Autodesk Inventor part; units mm, degrees
ref_plane "YZ Plane" through (0, 0, 0) normal (1, 0, 0) x (0, 1, 0)
ref_plane "XZ Plane" through (0, 0, 0) normal (0, 1, 0) x (-1, 0, 0)
ref_plane "XY Plane" through (0, 0, 0) normal (0, 0, 1) x (1, 0, 0)
sketch "Boceto1" plane through (0, 0, 0) normal (0, 1, 0) x (-1, 0, 0)
  line L0 (0, 0) -> (0, -2.6)
  line L1 (0, -2.6) -> (-2.7, -2.6)
  line L2 (-2.7, -2.6) -> (-2.7, -5.7)
  line L3 (-2.7, -5.7) -> (-12, -5.7)
  line L4 (-12, -5.7) -> (-12, -2.6)
  line L5 (-12, -2.6) -> (-14.7, -2.6)
  line L6 (-14.7, -2.6) -> (-14.7, 0)
  line L7 (-14.7, 0) -> (0, 0)
  line L8 (-12, -5.7) -> (-11.9, -5.7)
  line L9 (-11.9, -5.7) -> (-11.9, -2.6)
  line L10 (-11.9, -2.6) -> (-12, -2.6)
  line L11 (-12, -2.6) -> (-12, -5.7)
  line L12 (-2.7, -5.7) -> (-2.8, -5.7)
  line L13 (-2.8, -5.7) -> (-2.8, -2.6)
  line L14 (-2.8, -2.6) -> (-2.7, -2.6)
  line L15 (-2.7, -2.6) -> (-2.7, -5.7)
  line L16 (-2.7, -5.7) -> (4.75, -5.7)
  line L17 (-2.7, -5.7) -> (4.75, -5.7) construction
  line L18 (-12, -5.7) -> (-19.45, -5.7)
  line L19 (-12, -5.7) -> (-4.55, -5.7) construction
  line L20 (4.75, -5.7) -> (5.75, -5.7)
  line L21 (7.75, -7.7) -> (7.75, -8.7)
  line L22 (7.75, -8.7) -> (4.75, -8.7)
  line L23 (4.75, -8.7) -> (4.75, -5.7)
  line L24 (-19.45, -5.7) -> (-20.45, -5.7)
  line L25 (-22.45, -7.7) -> (-22.45, -8.7)
  line L26 (-22.45, -8.7) -> (-19.45, -8.7)
  line L27 (-19.45, -8.7) -> (-19.45, -5.7)
  line L28 (4.75, -8.7) -> (-19.45, -8.7)
  line L29 (4.75, -8.7) -> (7.75, -8.7)
  line L30 (7.75, -8.7) -> (7.75, -27.1)
  line L31 (7.75, -27.1) -> (4.75, -27.1)
  line L32 (4.75, -27.1) -> (4.75, -8.7)
  line L33 (-22.45, -8.7) -> (-19.45, -8.7)
  line L34 (-19.45, -8.7) -> (-19.45, -27.1)
  line L35 (-19.45, -27.1) -> (-22.45, -27.1)
  line L36 (-22.45, -27.1) -> (-22.45, -8.7)
  line L37 (7.75, -27.1) -> (-22.45, -27.1)
  line L38 (-22.45, -27.1) -> (-22.45, -28.1)
  line L39 (-20.45, -30.1) -> (5.75, -30.1)
  line L40 (7.75, -28.1) -> (7.75, -27.1)
  arc A0 (7.75, -7.7) -> (5.75, -5.7) centre (5.75, -7.7) ccw
  arc A1 (5.75, -30.1) -> (7.75, -28.1) centre (5.75, -28.1) ccw
  arc A2 (-22.45, -28.1) -> (-20.45, -30.1) centre (-20.45, -28.1) ccw
  arc A3 (-20.45, -5.7) -> (-22.45, -7.7) centre (-20.45, -7.7) ccw
  point P0 (-7.35, -5.7)
  point P1 (7.75, -5.7)
  point P2 (-22.45, -5.7)
  point P3 (-22.45, -30.1)
  point P4 (7.75, -30.1)
  dimension "d0" = 2.6
  dimension "d1" = 2.7
  dimension "d2" = 3.1
  dimension "d3" = 2.7
  dimension "d4" = 9.3
  dimension "d5" = 0.1
  dimension "d6" = 0.1
  dimension "d7" = 0
  dimension "d8" = 12.1
  dimension "d9" = 180
  dimension "d10" = 12.1
  dimension "d11" = 3
  dimension "d12" = 3
  dimension "d13" = 3
  dimension "d14" = 3
  dimension "d15" = 18.4
  dimension "d16" = 3
  dimension "d17" = 3
  dimension "d18" = 3
  dimension "d19" = 30.2
  dimension "d20" = 2
extrude "Extrusión1" add sketch "Boceto1" along normal blind 54.2 contours L0 L1 L14 L13 L3 L9 L10 L5 L6 L7 | L16 L23 L28 L27 L18 L3 | L20 A0 L21 L22 L23 | L22 L30 L31 L32 | L27 L26 L25 A3 L24 | L34 L35 L36 L26 | L31 L40 A1 L39 A2 L38 L35 L37
fillet "Empalme1" radius 1 20 edges at (-4.75, 54.2, -17.9) (-7.1642, 54.2, -29.5142) (-7.75, 54.2, -8.2) (-7.1642, 54.2, -6.2858) (2.75, 54.2, -5.7) (21.8642, 54.2, -29.5142) (22.45, 54.2, -8.2) (21.8642, 54.2, -6.2858) (11.95, 54.2, -5.7) (7.35, 54.2, -30.1) (7.35, 54.2, -27.1) (19.45, 54.2, -17.9) (7.35, 54.2, -8.7) (11.9, 54.2, -4.15) (2.8, 54.2, -4.15) (1.35, 54.2, -2.6) (0, 54.2, -1.3) (7.35, 54.2, 0) (14.7, 54.2, -1.3) (13.35, 54.2, -2.6)
properties part number "cajaBuck"
CAD build for the part. Positions are in the model's coordinates, mm. A direction names the side the tool comes from. Round coordinates to 2 decimals unless told otherwise and drop trailing zeros. Order: outer loops, then holes, each group sorted by start corner. A loop starts at its lowest first (then second) coordinate and runs counter-clockwise, first axis right, second up. Notation, with made-up numbers: (60.25, 88.5) - (103.25, 88.5) arc R25 cw to (103.25, 107.5) - close; hole circle Ø5 at (-11, 78.5). An arc over 180 degrees is marked (long way). Use CSV: the item, a comma, the result in double quotes. Start each with the question number.
1) Pin check, flat tips, straight feed: pin 1 Ø3.5 at (y, z) = (29, -3.5) entering from +X; pin 2 Ø1.3 at (y, z) = (39, -2) entering from -X; pin 3 Ø1.6 at (y, z) = (19.5, -4) entering from -X. Stop position of each tip, or through.
2) Tool access for faces 1 (the flat face through (19.45, 26, -18)), 2 (the flat face through (-2, 26, -5.7)), 3 (the flat face through (13, 26, -2.6)), 4 (the flat face through (14.7, 26, -1)), 5 (the flat face through (0, 26, -1)): list every direction of +Z, -Z, +X, -X, +Y, -Y with a clear straight run to the whole face (end or side of a thin tool).
3) Wall check: L1, parallel to Z at x = 1.5, y = 27; L2, parallel to X at y = 43.5, z = -16; L3, parallel to Z at x = -3, y = 48.5. Give the ranges that are in metal, low to high. Write a range as [from, to].
4) Saw through at D-D (x = 2). List the corners of the cut face in (y, z), and give its area (3 significant figures).
5) Saw through at C-C (y = 18). List the corners of the cut face in (x, z).
6) Saw through at B-B (z = -15). List the corners of the cut face in (x, y).
7) Two-plate mould, pull along Z, no slides. Class faces 6 (the cylindrical face through (-7.15, 26.23, -6.27)), 7 (the flat face through (16, 26, -5.7)), 8 (the flat face through (8, 26, -30.1)): pulls with the +Z half, pulls with the -Z half, needs draft (parallel to the pull), parting line crosses it, or undercut.
8) Saw through at A-A (x = -3.5). List the corners of the cut face in (y, z), and give its area (3 significant figures).
Values follow:
1,pin 1,"stops at x = 14.7"
1,pin 2,"stops at x = 0"
1,pin 3,"stops at x = 2.8"
2,face 1,"+Y, -Y"
2,face 2,"-X, +Y, -Y"
2,face 3,"+X, +Y, -Y"
2,face 4,"+Z, +X, +Y, -Y"
2,face 5,"+Z, -X, +Y, -Y"
3,L1,"z = [-30.1, -27.1], [-8.7, -5.7], [-2.6, 0]"
3,L2,"x = [-7.75, -4.75], [19.45, 22.45]"
3,L3,"z = [-30.1, -27.1], [-8.7, -5.7]"
4,outline,"(0, -30.1) - (53.2, -30.1) arc R1 ccw to (54.2, -29.1) - (54.2, -28.1) arc R1 ccw to (53.2, -27.1) - (0, -27.1) - close; (0, -8.7) - (53.2, -8.7) arc R1 ccw to (54.2, -7.7) - (54.2, -6.7) arc R1 ccw to (53.2, -5.7) - (0, -5.7) - close; (0, -2.6) - (53.2, -2.6) arc R1 ccw to (54.2, -1.6) - (54.2, -1) arc R1 ccw to (53.2, 0) - (0, 0) - close"
4,area,"465 mm2"
5,outline,"(-7.75, -28.1) arc R2 ccw to (-5.75, -30.1) - (20.45, -30.1) arc R2 ccw to (22.45, -28.1) - (22.45, -7.7) arc R2 ccw to (20.45, -5.7) - (11.9, -5.7) - (11.9, -2.6) - (14.7, -2.6) - (14.7, 0) - (0, 0) - (0, -2.6) - (2.8, -2.6) - (2.8, -5.7) - (-5.75, -5.7) arc R2 ccw to (-7.75, -7.7) - close; hole (-4.75, -27.1) - (19.45, -27.1) - (19.45, -8.7) - (-4.75, -8.7) - close"
6,outline,"(-7.75, 0) - (-4.75, 0) - (-4.75, 53.2) arc R1 ccw to (-5.75, 54.2) - (-6.75, 54.2) arc R1 ccw to (-7.75, 53.2) - close; (19.45, 0) - (22.45, 0) - (22.45, 53.2) arc R1 ccw to (21.45, 54.2) - (20.45, 54.2) arc R1 ccw to (19.45, 53.2) - close"
7,face 6,"pulls with the +Z half"
7,face 7,"undercut"
7,face 8,"pulls with the -Z half"
8,outline,"(0, -30.1) - (53.2, -30.1) arc R1 ccw to (54.2, -29.1) - (54.2, -28.1) arc R1 ccw to (53.2, -27.1) - (0, -27.1) - close; (0, -8.7) - (53.2, -8.7) arc R1 ccw to (54.2, -7.7) - (54.2, -6.7) arc R1 ccw to (53.2, -5.7) - (0, -5.7) - close"
8,area,"324 mm2"
